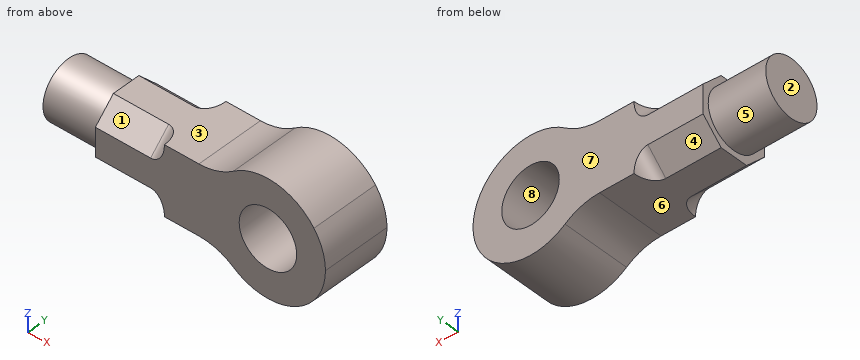
from build123d import *

# Parameters (mm, degrees)
SKETCH1_W           = 200
SKETCH1_H           = 60
BOSS_EXTRUDE1_DEPTH = 60
SKETCH2_R           = 50
SKETCH2_R_2         = 25
BOSS_EXTRUDE2_DEPTH = 60
SKETCH3_R           = 25
CUT_EXTRUDE1_DEPTH  = 60
SKETCH4_R           = 25
BOSS_EXTRUDE3_DEPTH = 50
CUT_EXTRUDE2_DEPTH  = 60
FILLET1_R           = 12
FILLET2_R           = 50


with BuildPart() as part:
    # Sketch1 → Boss-Extrude1 (new body)
    with BuildSketch(Plane.XY):
        with Locations((-100, 30)):
            Rectangle(SKETCH1_W, SKETCH1_H)
    extrude(amount=BOSS_EXTRUDE1_DEPTH)

    # Sketch2 → Boss-Extrude2 (add)
    with BuildSketch(Plane(origin=(0, 60, 0), x_dir=(1, 0, 0), z_dir=(0, 1, 0))):
        with Locations((-50, -30)):
            Circle(SKETCH2_R)
        with Locations((-50, -30)):
            Circle(SKETCH2_R_2, mode=Mode.SUBTRACT)
    extrude(amount=-BOSS_EXTRUDE2_DEPTH)

    # Sketch3 → Cut-Extrude1 (cut)
    with BuildSketch(Plane(origin=(0, 60, 0), x_dir=(1, 0, 0), z_dir=(0, 1, 0))):
        with Locations(Location((-50, -30, 0), (0, 0, 180))):
            Circle(SKETCH3_R)
        with BuildLine():
            ThreePointArc((-10, 0), (-2.565835097, -14.188611699), (0, -30))
            Line((0, -30), (0, 0))
            Line((0, 0), (-10, 0))
        make_face()
        with BuildLine():
            Line((-10, -60), (0, -60))
            Line((0, -60), (0, -30))
            ThreePointArc((0, -30), (-2.565835097, -45.811388301), (-10, -60))
        make_face()
    extrude(amount=-CUT_EXTRUDE1_DEPTH, mode=Mode.SUBTRACT)

    # Sketch4 → Boss-Extrude3 (add)
    with BuildSketch(Plane.ZY.offset(200)):
        with Locations(Location((30, 30, 0), (0, 0, 180))):
            Circle(SKETCH4_R)
    extrude(amount=BOSS_EXTRUDE3_DEPTH)

    # Sketch5 → Cut-Extrude2 (cut)
    with BuildSketch(Plane.ZY.offset(200)):
        Polygon((60, 60), (42.426406871, 60), (60, 42.426406871), align=None)
        Polygon((0, 42.426406871), (17.573593129, 60), (0, 60), align=None)
        Polygon((17.573593129, 0), (0, 17.573593129), (0, 0), align=None)
        Polygon((60, 0), (60, 17.573593129), (42.426406871, 0), align=None)
    extrude(amount=-CUT_EXTRUDE2_DEPTH, mode=Mode.SUBTRACT)

    # Fillet1
    fillet1_edges = [part.edges().sort_by_distance(p)[0] for p in [
        (-140, 8.786796564, 51.213203436),
        (-140, 51.213203436, 51.213203436),
        (-140, 51.213203436, 8.786796564),
        (-140, 8.786796564, 8.786796564),
    ]]
    fillet(fillet1_edges, radius=FILLET1_R)

    # Fillet2
    fillet2_edges = [part.edges().sort_by_distance(p)[0] for p in [
        (-90, 30, 0),
        (-90, 30, 60),
    ]]
    fillet(fillet2_edges, radius=FILLET2_R)


solid = part.part
Geometry check sheet. Reference: the model listing, model coordinates, mm. Face numbers are marked on the shaded views. A direction names the side the tool comes from. Coordinates: 2 decimals unless noted, no trailing zeros. Write each loop counter-clockwise with the first axis right and the second up, starting at its lowest first coordinate (ties: lowest second). Pieces come first, ordered by that corner, then holes. Notation, with made-up numbers: (44, 19) -> (71, 19) arc R16 cw to (71, 42) -> close; hole circle Ø8 at (86.5, 22.5). An arc over 180 degrees is marked (long way). One line per question, with ' | ' between items.
1. Depth check by flat-ended pin: pin 1 Ø10 at (y, z) = (32.5, 52) entering from +X; pin 2 Ø18 at (x, y) = (-146, 36.5) entering from -Z; pin 3 Ø1.5 at (x, y) = (-31.5, 18) entering from -Z. Enter the tip coordinate at first touch or a pass-through.
Answers:
pin 1: stops at x = -2.98 | pin 2: stops at z = 0 | pin 3: stops at z = -16.74
2. Cross-section at D-D on x = -131. Record the cut outline in (y, z), and give its area (3 significant figures).
Answers:
outline: (0, 0) -> (60, 0) -> (60, 60) -> (0, 60) -> close | area: 3,600 mm²
3. Cross-section at C-C on x = -211.5. Record the cut outline in (y, z), and give its area (3 significant figures).
Answers:
outline: circle Ø50 at (30, 30) | area: 1,960 mm²
4. Set-up check for the marked faces 1, 2, 3, 4 and 5: record each of +Z, -Z, +X, -X, +Y, -Y from which the full face is reachable in a straight line by a thin tool's end or side.
Answers:
face 1: +Z, -X, -Y | face 2: +Z, -Z, -X, +Y, -Y | face 3: +Z, -X, +Y, -Y | face 4: -Z, -X, +Y | face 5: -X
5. Draft check along Z on the marked faces 6, 7 and 8. Enter one of: +Z half, -Z half, draft (parallel to the pull), parting line (faces both ways), or undercut.
Answers:
face 6: -Z half | face 7: draft | face 8: undercut
6. Thickness scan on probe 1 along Z at (x, y) = (-50, 21); probe 2 along X at (y, z) = (39, 29); probe 3 along X at (y, z) = (43.5, 19.5). Record the ranges inside material, lowest first. Write a range as from..to.
Answers:
probe 1: z = -20..5, 55..80 | probe 2: x = -250..-74.98, -25.02..-0.01 | probe 3: x = -250..-72.69, -27.31..-1.11
7. Cross-section at A-A on x = -50. Record the cut outline in (y, z), and give its area (3 significant figures).
Answers:
outline: (0, -20) -> (60, -20) -> (60, 5) -> (0, 5) -> close; (0, 55) -> (60, 55) -> (60, 80) -> (0, 80) -> close | area: 3,000 mm²
8. Cross-section at B-B on y = 30. Record the cut outline in (x, z), and give its area (3 significant figures).
Answers:
outline: (-250, 5) -> (-200, 5) -> (-200, 0) -> (-110, 0) arc R50 cw to (-80, -10) arc R50 ccw (long way) to (-80, 70) arc R50 cw to (-110, 60) -> (-200, 60) -> (-200, 55) -> (-250, 55) -> close; hole circle Ø50 at (-50, 30) | area: 14,700 mm²
